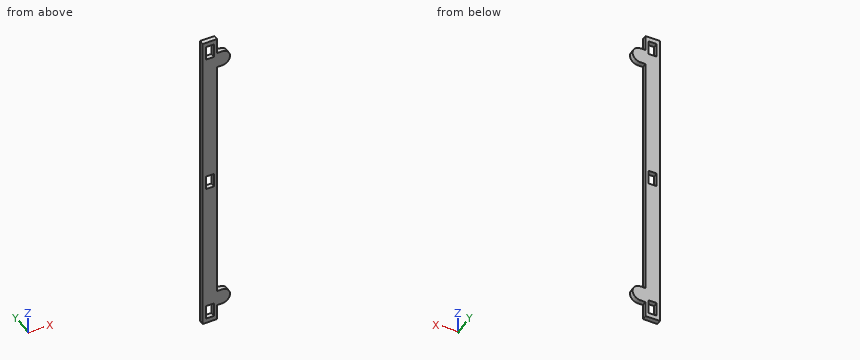
Autodesk Inventor part; units mm, degrees
ref_plane "YZ Plane" through (0, 0, 0) normal (1, 0, 0) x (0, 1, 0)
ref_plane "XZ Plane" through (0, 0, 0) normal (0, 1, 0) x (-1, 0, 0)
ref_plane "XY Plane" through (0, 0, 0) normal (0, 0, 1) x (1, 0, 0)
sketch "草圖1" plane through (0, 0, 0) normal (0, 1, 0) x (-1, 0, 0)
  line L0 (0, 80) -> (9, 80)
  line L1 (9, 80) -> (9, -80)
  line L2 (9, -80) -> (0, -80)
  line L3 (0, -80) -> (0, 80)
  line L4 (7, 4.5) -> (2, 4.5)
  line L5 (2, 4.5) -> (2, -4.5)
  line L6 (2, -4.5) -> (7, -4.5)
  line L7 (7, -4.5) -> (7, 4.5)
  line L8 (9, 80) -> (9, 90)
  line L9 (9, 90) -> (-3, 90)
  line L10 (-8, 85) -> (-8, 85)
  line L11 (-3, 80) -> (0, 80)
  arc A0 (-8, 85) -> (-3, 80) centre (-3, 85) ccw
  arc A1 (-3, 90) -> (-8, 85) centre (-3, 85) ccw
  circle A2 centre (-3, 85) radius 2.5
  line L12 (9, 0) -> (0, 0)
  line L13 (9, -80) -> (9, -90)
  line L14 (9, -90) -> (-3, -90)
  line L15 (-3, -80) -> (0, -80)
  arc A3 (-3, -80) -> (-8, -85) centre (-3, -85) ccw
  arc A4 (-8, -85) -> (-3, -90) centre (-3, -85) ccw
  circle A5 centre (-3, -85) radius 2.5
  line L16 (9, 90) -> (0, 90)
  line L17 (0, 90) -> (0, 100)
  line L18 (0, 100) -> (9, 100)
  line L19 (9, 100) -> (9, 90)
  line L20 (9, -90) -> (0, -90)
  line L21 (0, -90) -> (0, -100)
  line L22 (0, -100) -> (9, -100)
  line L23 (9, -100) -> (9, -90)
  line L24 (7, 97) -> (2, 97)
  line L25 (2, 97) -> (2, 88)
  line L26 (2, 88) -> (7, 88)
  line L27 (7, 88) -> (7, 97)
  line L28 (7, -97) -> (2, -97)
  line L29 (2, -97) -> (2, -88)
  line L30 (2, -88) -> (7, -88)
  line L31 (7, -88) -> (7, -97)
  point P0 (7, 0)
  point P1 (4.5, 4.5)
  point P2 (4.5, 80)
  point P3 (-8, 90)
  point P4 (-8, -90)
  point P5 (-8, -85)
  point P6 (4.5, 97)
  point P7 (4.5, 100)
  point P8 (4.5, -97)
  dimension "d0" = 160
  dimension "d1" = 9
  dimension "d2" = 9
  dimension "d3" = 5
  dimension "d4" = 10
  dimension "d5" = 17
  dimension "d6" = 5
  dimension "d7" = 5
  dimension "d8" = 5
  dimension "d11" = 9
  dimension "d12" = 10
  dimension "d13" = 10
  dimension "d14" = 9
  dimension "d15" = 5
  dimension "d16" = 9
  dimension "d17" = 3
extrude "擠出1" add sketch "草圖1" along normal blind 3 contours L11 A0 A1 L9 L25 L26 L27 L8 L0 | L0 L1 L12 L7 L4 L5 L3 | L12 L5 L6 L7 L1 L2 L3 | L9 L27 L24 L25 L17 L18 L19 | L2 L13 L14 L31 L30 L29 A4 A3 L15 | L23 L22 L21 L14 L29 L28 L31 | A2 | A5
properties part number "upper_Bar_3" material "木材 (樺木)"
Read the model definition and answer for the solid it produces. Units are mm, in the model's axes. Coordinates: 2 decimals unless noted, no trailing zeros. Write each loop counter-clockwise with the first axis right and the second up, starting at its lowest first coordinate (ties: lowest second). Pieces come first, ordered by that corner, then holes. Notation, with made-up numbers: (14, -17) -> (23, -17) arc R17 cw to (23, -8) -> close; hole circle Ø7 at (-6.5, 32). An arc over 180 degrees is marked (long way). Answer as a JSON object with one key per item and string values.
Q1. The part is cut by section B-B on z = 57. Give the vertices of the cut face in (x, y).
The answers:
{"outline": "(-9, 0) -> (0, 0) -> (0, 3) -> (-9, 3) -> close"}
Q2. Flat-ended cylindrical pins translate along their axes: pin 1 Ø1.5 at (y, z) = (2, 1.5) entering from +X; pin 2 Ø0.9 at (x, y) = (2, 1.5) entering from -Z. Find the tip coordinate at first contact, or state that the pin passes through.
The answers:
{"pin 1": "stops at x = 0", "pin 2": "stops at z = -90"}
Q3. The part is cut by section C-C on z = 82.5. Give the vertices of the cut face in (x, y).
The answers:
{"outline": "(-9, 0) -> (7.33, 0) -> (7.33, 3) -> (-9, 3) -> close"}
Q4. Consider line 1 (Z direction, x = -4.75, y = 0.65); line 2 (Z direction, x = 3.5, y = 2.3); line 3 (X direction, y = 1.9, z = -2.5). Determine where each line is inside the solid, lowest interval first. Write a range as [from, to].
The answers:
{"line 1": "z = [-100, -97], [-88, -4.5], [4.5, 88], [97, 100]", "line 2": "z = [-89.97, -80.03], [80.03, 89.97]", "line 3": "x = [-9, -7], [-2, 0]"}
Q5. The part is cut by section A-A on y = 0.6. Give the vertices of the cut face in (x, z), then the cut area to 3 significant figures.
The answers:
{"outline": "(-9, -100) -> (0, -100) -> (0, -90) -> (3, -90) arc R5 ccw to (3, -80) -> (0, -80) -> (0, 80) -> (3, 80) arc R5 ccw to (3, 90) -> (0, 90) -> (0, 100) -> (-9, 100) -> close; hole (-7, -97) -> (-2, -97) -> (-2, -88) -> (-7, -88) -> close; hole (-7, -4.5) -> (-2, -4.5) -> (-2, 4.5) -> (-7, 4.5) -> close; hole (-7, 88) -> (-2, 88) -> (-2, 97) -> (-7, 97) -> close", "area": "1,800 mm2"}
